```python
from build123d import *

# Parameters (mm, degrees)
F1_DEPTH = 139.7
F2_T     = -2.54
F3_W     = 304.8
F3_H     = 342.9
F4_DEPTH = 2.54


with BuildPart() as f1:
    # F0 (on Top) → F1 (new body, symmetric)
    with BuildSketch(Plane.XY):
        Polygon((-152.4, 342.9), (-292.1, 0), (292.1, 0), (152.4, 342.9), align=None)
    extrude(amount=F1_DEPTH, both=True)

    # F2
    f2_openings = [f1.faces().sort_by_distance(p)[0] for p in [
        (0, 0, 0),
    ]]
    offset(amount=F2_T, openings=f2_openings)

    # F3 (on face) → F4 (cut, through all)
    with BuildSketch(Plane.XY.offset(139.7)):
        with Locations((0, 171.45)):
            Rectangle(F3_W, F3_H)
    extrude(amount=-F4_DEPTH, mode=Mode.SUBTRACT)


solid = f1.part
```
Model file for the job. Use its own axes, mm. A direction names the side the tool comes from. Coordinates: 2 decimals unless noted, no trailing zeros. Loops run counter-clockwise (first coordinate to the right, second up) from the corner with the lowest first, then second, coordinate; pieces in that order, holes last. Notation, with made-up numbers: (72, 81.25) - (128, 81.25) arc R33 cw to (128, 115.25) - close; hole circle Ø9 at (22, 73.5). An arc over 180 degrees is marked (long way). Answer as a JSON object with one key per item and string values. Group by question number.
(1) Flat gauge pins, fed straight in: pin 1 (1.5 mm diameter, centred on x = -231, z = -12, fed in from -Y); pin 2 (10 mm diameter, centred on y = 111, z = -107.5, fed in from -X); pin 3 (4 mm diameter, centred on x = 57.5, y = 231.5, fed in from +Z). Where does each tip first touch, or does it go through?
(2) Probe line 1 along Z through (x, y) = (169, 236); line 2 along Z through (x, y) = (-75, 175); line 3 along Y through (x, z) = (-109, 9). List the from-to ranges inside material, lowest first.
(3) Cut at C-C (y = 171). Give the cut face in (x, z), then the cut area to 3 significant figures.
(4) Tool access for faces 4 (the face through (220.995, 167.797, 1.92)), 5 (the face through (223.228, 169.05, 1.956)), 6 (the face through (2, 340.36, 2)): list every direction of +Z, -Z, +X, -X, +Y, -Y with a clear straight run to the whole face (end or side of a thin tool).
(5) Cut at B-B (x = 78). Give the cut face in (y, z), then the cut area to 3 significant figures.
(6) Two-plate mould, pull along Z, no slides. Class faces 1 (the face through (-191, 96, 137.16)), 2 (the face through (190, 98, 139.7)), 3 (the face through (-4, 136, -139.7)): released by +Z, released by -Z, zero draft, split by the parting line, or undercut.
(7) Cut at D-D (x = 227). Give the cut face in (y, z), then the cut area to 3 significant figures.
(8) Cut at A-A (z = 43). Give the cut face in (x, y).
Geometry says:
{
 "1": {"pin 1": "stops at y = 141.4", "pin 2": "stops at x = -248.91", "pin 3": "stops at z = -137.16"},
 "2": {"line 1": "z = -139.7 to -137.16, 137.16 to 139.7", "line 2": "z = -139.7 to -137.16", "line 3": "y = 340.36 to 342.9"},
 "3": {"outline": "(-222.43, -139.7) - (222.43, -139.7) - (222.43, 139.7) - (152.4, 139.7) - (152.4, 137.16) - (219.69, 137.16) - (219.69, -137.16) - (-219.69, -137.16) - (-219.69, 137.16) - (-152.4, 137.16) - (-152.4, 139.7) - (-222.43, 139.7) - close", "area": "2,990 mm^2"},
 "4": {"face 4": "-Y", "face 5": "+Z, -Z, +X, +Y", "face 6": "+Z, -Y"},
 "5": {"outline": "(0, -139.7) - (342.9, -139.7) - (342.9, 137.16) - (340.36, 137.16) - (340.36, -137.16) - (0, -137.16) - close", "area": "1,570 mm^2"},
 "6": {"face 1": "undercut", "face 2": "released by +Z", "face 3": "released by -Z"},
 "7": {"outline": "(0, -139.7) - (159.79, -139.7) - (159.79, 139.7) - (0, 139.7) - (0, 137.16) - (153.06, 137.16) - (153.06, -137.16) - (0, -137.16) - close", "area": "2,660 mm^2"},
 "8": {"outline": "(-292.1, 0) - (-289.36, 0) - (-150.69, 340.36) - (150.69, 340.36) - (289.36, 0) - (292.1, 0) - (152.4, 342.9) - (-152.4, 342.9) - close"}
}
